```python
from build123d import *

# Parameters (mm, degrees)
BOSS_EXTRUDE1_DEPTH = 92
FILLET1_R           = 3
SKETCH2_R           = 3.25
CUT_EXTRUDE1_DEPTH  = 92


with BuildPart() as part:
    # Sketch1 → Boss-Extrude1 (new body)
    with BuildSketch(Plane(origin=(0, 0, 0), x_dir=(1, 0, 0), z_dir=(0, 1, 0))):
        Polygon((-4, 5), (-4, 13), (4, 13), (4, 5), (20, 5), (20, 0), (-20, 0), (-20, 5), align=None)
    extrude(amount=-BOSS_EXTRUDE1_DEPTH)

    # Fillet1
    fillet1_edges = [part.edges().sort_by_distance(p)[0] for p in [
        (-4, -46, -5),
        (4, -46, -5),
    ]]
    fillet(fillet1_edges, radius=FILLET1_R)

    # Sketch2 → Cut-Extrude1 (cut)
    with BuildSketch(Plane.XY):
        with Locations((12.5, -8)):
            Circle(SKETCH2_R)
        with Locations((12.5, -33)):
            Circle(SKETCH2_R)
        with Locations((-12.5, -33)):
            Circle(SKETCH2_R)
        with Locations((-12.5, -8)):
            Circle(SKETCH2_R)
    extrude(amount=-CUT_EXTRUDE1_DEPTH, mode=Mode.SUBTRACT)


solid = part.part
```
The model under review builds one solid part; all positions refer to its coordinate system, in mm. A direction names the side the tool comes from. Round coordinates to 2 decimals unless told otherwise and drop trailing zeros. Loops run counter-clockwise (first coordinate to the right, second up) from the corner with the lowest first, then second, coordinate; pieces in that order, holes last. Notation, with made-up numbers: (87, -27.75) - (132, -27.75) arc R25 cw to (132, -5.75) - close; hole circle Ø8 at (-28.5, 86). An arc over 180 degrees is marked (long way). Write each question's results on one line, items separated by ' | '. Start each with the question number.
Q1. Take a section at A-A on x = -12.5. Give the boundary of the cut face in (y, z), plus the area to 3 significant figures.
Q2. Take a section at D-D on z = -2.25. Give the boundary of the cut face in (x, y).
Q3. Take a section at B-B on y = -8. Give the boundary of the cut face in (x, z).
Q4. Wall thickness on line 1 along Y through (x, z) = (12.5, -1.3); line 2 along X through (y, z) = (-27, -11.5); line 3 along Z through (x, y) = (-7, -42): over which ranges is each line inside the solid? List them lowest first. Write a range as [from, to].
Q5. Draft analysis for pull direction X (two halves, no side actions). For faces 1 (the flat face through (-20, -45, -2)), 2 (the cylindrical face through (11.795, -36.173, -2.465)), 3 (the flat face through (20, -45, -3)), 4 (the flat face through (0, -45, -13)), state which applies: pulls with the +X half, pulls with the -X half, needs draft (parallel to the pull), parting line crosses it, or undercut.
Q6. Tool access review of faces 5 (the flat face through (4, -45, -11)), 6 (the flat face through (-4, -45, -10)), 7 (the flat face through (0, -45, 0)): name each direction out of +Z, -Z, +X, -X, +Y, -Y from which nothing blocks a thin tool from reaching the whole face with its end or side.
Q7. Take a section at C-C on y = -47. Give the boundary of the cut face in (x, z).
Q8. Insertion check: P1, Ø3, axis at y = -25.5, z = -7.5, coming from the +X side; P2, Ø7.5, axis at x = 12.5, y = -8, coming from the -Z side; P3, Ø5.5, axis at y = -36, z = -9.5, coming from the +X side. Each pin has a flat end and moves straight along its axis. Give the tip position at first contact, or say it passes through.
Data:
1) outline: (-92, -5) - (-36.25, -5) - (-36.25, 0) - (-92, 0) - close; (-29.75, -5) - (-11.25, -5) - (-11.25, 0) - (-29.75, 0) - close; (-4.75, -5) - (0, -5) - (0, 0) - (-4.75, 0) - close | area: 395 mm²
2) outline: (-20, -92) - (20, -92) - (20, 0) - (-20, 0) - close; hole circle Ø6.5 at (-12.5, -33); hole circle Ø6.5 at (-12.5, -8); hole circle Ø6.5 at (12.5, -33); hole circle Ø6.5 at (12.5, -8)
3) outline: (-20, -5) - (-15.75, -5) - (-15.75, 0) - (-20, 0) - close; (-9.25, -5) - (-7, -5) arc R3 cw to (-4, -8) - (-4, -13) - (4, -13) - (4, -8) arc R3 cw to (7, -5) - (9.25, -5) - (9.25, 0) - (-9.25, 0) - close; (15.75, -5) - (20, -5) - (20, 0) - (15.75, 0) - close
4) line 1: y = [-92, -36.25], [-29.75, -11.25], [-4.75, 0] | line 2: x = [-4, 4] | line 3: z = [-5, 0]
5) face 1: pulls with the -X half | face 2: undercut | face 3: pulls with the +X half | face 4: needs draft
6) face 5: -Z, +X, +Y, -Y | face 6: -Z, -X, +Y, -Y | face 7: +Z, +X, -X, +Y, -Y
7) outline: (-20, -5) - (-7, -5) arc R3 cw to (-4, -8) - (-4, -13) - (4, -13) - (4, -8) arc R3 cw to (7, -5) - (20, -5) - (20, 0) - (-20, 0) - close
8) P1: stops at x = 4.76 | P2: stops at z = -5 | P3: stops at x = 4.27
